The listing builds one solid part. Answer for the finished solid, in the listing's coordinates (mm). Face numbers are marked on the shaded views. A direction names the side the tool comes from. Give positions to 0.01 mm unless a question says otherwise; leave off trailing zeros. Loops run counter-clockwise (first coordinate to the right, second up) from the corner with the lowest first, then second, coordinate; pieces in that order, holes last. Notation, with made-up numbers: (2, 21) - (55, 21) arc R31 ccw to (55, 48) - close; hole circle Ø8 at (5.25, 37). An arc over 180 degrees is marked (long way). One line per item, written item: value. Start each with the question number.
Autodesk Inventor part; units mm, degrees
ref_plane "YZ Plane" through (0, 0, 0) normal (1, 0, 0) x (0, 1, 0)
ref_plane "XZ Plane" through (0, 0, 0) normal (0, 1, 0) x (-1, 0, 0)
ref_plane "XY Plane" through (0, 0, 0) normal (0, 0, 1) x (1, 0, 0)
sketch "Esquisse1" plane through (0, 0, 0) normal (0, 1, 0) x (-1, 0, 0)
  circle A0 centre (0, 0) radius 3
  dimension "d0" = 6
extrude "Extrusion1" add sketch "Esquisse1" along normal blind 100
sketch "Esquisse2" plane through (0, 0, 0) normal (0, -1, 0) x (1, 0, 0)
  circle A0 centre (0, 0) radius 3
  circle A1 centre (0, 0) radius 5
  dimension "d3" = 10
extrude "Extrusion2" add sketch "Esquisse2" along normal blind 2 contours A0 | A1
fillet "Congé1" radius 2 1 edges at (-5, -2, 0)
properties part number "vis_6mm_100mm"
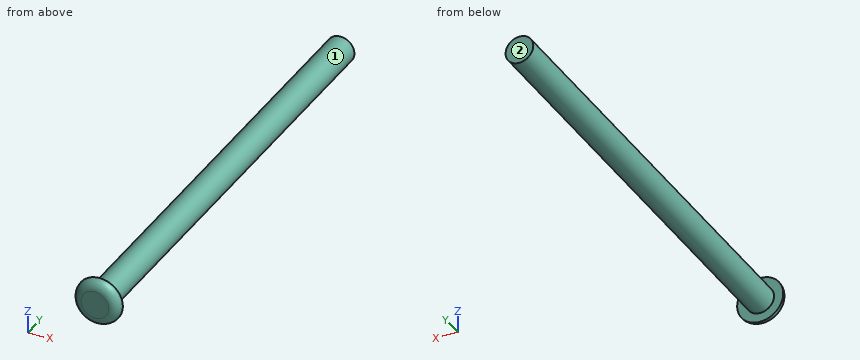
1. Find the intervals of material crossed by L1, parallel to Y at x = 1.25, z = 3; L2, parallel to Z at x = 0.25, y = 36.5; L3, parallel to X at y = 48, z = 0.5, in increasing order. Write a range as [from, to].
2. A cutting plane is placed at C-C (y = 26). Determine the outline of the cut face in (x, z), plus the area to 3 significant figures.
3. Flat-ended cylindrical pins translate along their axes: pin 1 (5 mm diameter, centred on x = -4, y = 86, fed in from -Z); pin 2 (4 mm diameter, centred on x = -1.5, y = 65.5, fed in from -Z); pin 3 (1.5 mm diameter, centred on y = 78, z = 3, fed in from +X). Find the tip coordinate at first contact, or state that the pin passes through.
4. For the marked faces 1 and 2, determine the directions among +Z, -Z, +X, -X, +Y, -Y from which every point of the face is accessible in a straight line to the end or side of a thin tool.
Results below:
1. L1: y = [-1.98, 0]
1. L2: z = [-2.99, 2.99]
1. L3: x = [-2.96, 2.96]
2. outline: circle Ø6 at (0, 0)
2. area: 28.3 mm^2
3. pin 1: stops at z = -2.6
3. pin 2: stops at z = -3
3. pin 3: stops at x = 1.98
4. face 1: +Y
4. face 2: +Z, -Z, +X, -X, +Y
